Can you work these out from the model? Positions are in its coordinate system, mm. Face numbers are marked on the shaded views. A direction names the side the tool comes from. Round coordinates to 2 decimals unless told otherwise and drop trailing zeros. Write each loop counter-clockwise with the first axis right and the second up, starting at its lowest first coordinate (ties: lowest second). Pieces come first, ordered by that corner, then holes. Notation, with made-up numbers: (75.5, -33.75) - (92.5, -33.75) arc R17 cw to (92.5, -24.75) - close; hole circle Ø10 at (-12, 61). An arc over 180 degrees is marked (long way). One line per item, written item: value. Start each with the question number.
(1) I want a section at C-C on x = 24.5. List the corners of the cut face in (y, z) for me.
(2) On a 3-axis mill with a long thin cutter (end or side, diameter ignored), from which of +Z, -Z, +X, -X, +Y, -Y can I reach the whole of each face in a straight line? I mean the marked faces 1 and 2. Say none if no direction works.
(3) I'm going to push flat-ended pins straight in: pin 1 Ø8 at (x, z) = (33, -5) entering from -Y; pin 2 Ø2 at (x, z) = (-2, 0) entering from -Y; pin 3 Ø2 at (y, z) = (72, -6) entering from +X; pin 4 Ø10 at (y, z) = (-5, 3) entering from +X. Where does each tip first touch, or does it pass through?
(4) If I drill on L1, parallel to X at y = 0, z = 1.5; L2, parallel to Y at x = 18, z = -2.5; L3, parallel to Y at x = 14, z = 5.5, over which ranges is the centre line in solid material (lowest first)? Write a range as from..to.
(5) Thinking about a two-plate mould opening in Y: for the marked faces 3, 4 and 5, which applies, +Y half, -Y half, draft (parallel to the pull), parting line (faces both ways), or undercut?
(6) I want a section at B-B on y = 0. List the corners of the cut face in (x, z) for me.
(7) I want a section at A-A on z = -5.25. List the corners of the cut face in (x, y) for me, plus the area to 3 significant figures.
from build123d import *

# Parameters (mm, degrees)
SKETCH_3_W = 3
SKETCH_3_H = 20


with BuildPart() as part:
    # 扫描1: sweep along a path in 草图2
    with BuildLine(Plane.XY) as sweep_1_path:
        Line((-56.997873172, 6.020936707), (-47.843990191, 92.677197452))
        ThreePointArc((-47.843990191, 92.677197452), (-28.681020404, 114.724081616), (-1.397513338, 104.288816665))
        Line((-1.397513338, 104.288816665), (47.458859055, 32.135119764))
        ThreePointArc((47.458859055, 32.135119764), (13.900929349, -55.603717396), (-56.997873172, 6.020936707))
    # 草图3 → 扫描1 (sweep)
    with BuildSketch(Plane(origin=(0, 0, 0), x_dir=(1, 0, 0), z_dir=(0, 1, 0))):
        with Locations((-56.5, 0)):
            Rectangle(SKETCH_3_W, SKETCH_3_H)
    sweep(path=sweep_1_path.line)


solid = part.part
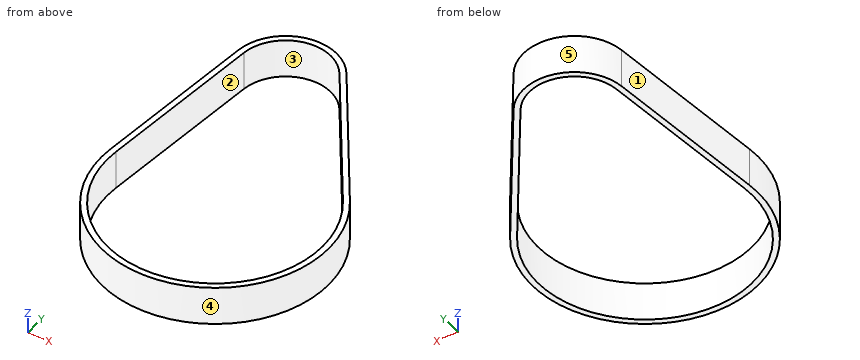
Established:
1. outline: (-52.57, -10) - (-49.24, -10) - (-49.24, 10) - (-52.57, 10) - close; (61.91, -10) - (67.26, -10) - (67.26, 10) - (61.91, 10) - close
2. face 1: +Z, -Z, -X, +Y
2. face 2: +Z, -Z
3. pin 1: y = -50.23
3. pin 2: y = -57.99
3. pin 3: x = 21.97
3. pin 4: x = 58
4. L1: -58..-55, 55..58
4. L2: -55.14..-51.97, 71.51..76.86
4. L3: -56.28..-53.19, 77.42..82.77
5. face 3: undercut
5. face 4: parting line
5. face 5: +Y half
6. outline: (-58, -10) - (-55, -10) - (-55, 10) - (-58, 10) - close; (55, -10) - (58, -10) - (58, 10) - (55, 10) - close
7. outline: (-57.68, 6.09) arc R58 ccw (long way) to (48.03, 32.52) - (-0.83, 104.67) arc R26.17 ccw to (-48.53, 92.75) - close; hole (-54.7, 5.78) arc R55 ccw (long way) to (45.54, 30.84) - (-3.31, 102.99) arc R23.17 ccw to (-45.54, 92.43) - close
7. area: 1,350 mm2
